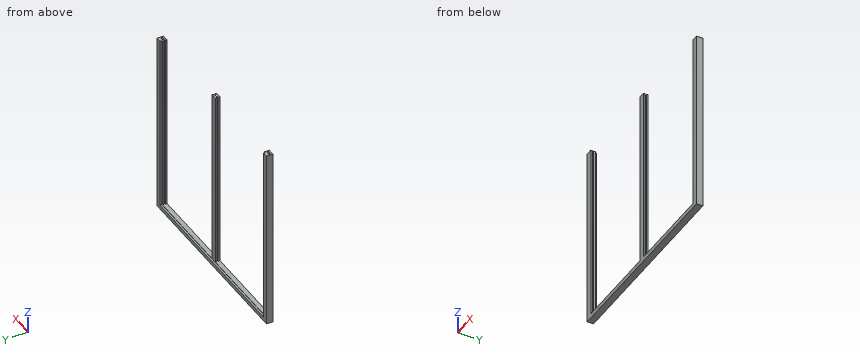
```python
from build123d import *

# Parameters (mm, degrees)
SKETCH1_W           = 2.25
SKETCH1_H           = 1.45
BOSS_EXTRUDE1_DEPTH = 5
BOSS_EXTRUDE2_DEPTH = 200
BOSS_EXTRUDE3_DEPTH = 2
SKETCH4_W           = 2
SKETCH4_H           = 2
CUT_EXTRUDE1_DEPTH  = 3


with BuildPart() as part:
    # Sketch1 → Boss-Extrude1 (new body)
    with BuildSketch(Plane.XY):
        Polygon((0, 0), (7, 0), (7, 1.775), (4.75, 1.775), (4.75, 3.225), (7, 3.225), (7, 5), (0, 5), align=None)
        with Locations((5.875, 2.5)):
            Rectangle(SKETCH1_W, SKETCH1_H)
        Polygon((7, 0), (102.75, 0), (102.75, 1.775), (102.75, 3.225), (102.75, 5), (7, 5), (7, 3.225), (7, 1.775), align=None)
        with Locations((103.875, 2.5)):
            Rectangle(SKETCH1_W, SKETCH1_H)
        Polygon((102.75, 0), (106, 0), (106, 5), (102.75, 5), (102.75, 3.225), (105, 3.225), (105, 1.775), (102.75, 1.775), align=None)
        Polygon((106, 5), (106, 0), (109.25, 0), (109.25, 1.775), (107, 1.775), (107, 3.225), (109.25, 3.225), (109.25, 5), align=None)
        with Locations((108.125, 2.5)):
            Rectangle(SKETCH1_W, SKETCH1_H)
        Polygon((109.25, 1.775), (109.25, 0), (205, 0), (205, 1.775), (205, 3.225), (205, 5), (109.25, 5), (109.25, 3.225), align=None)
        with Locations((206.125, 2.5)):
            Rectangle(SKETCH1_W, SKETCH1_H)
        Polygon((205, 1.775), (205, 0), (212, 0), (212, 5), (205, 5), (205, 3.225), (207.25, 3.225), (207.25, 1.775), align=None)
    extrude(amount=BOSS_EXTRUDE1_DEPTH)

    # Sketch2 → Boss-Extrude2 (add)
    with BuildSketch(Plane.XY.offset(5)):
        Polygon((7, 3.225), (7, 5), (0, 5), (0, 0), (7, 0), (7, 1.775), (4.75, 1.775), (4.75, 3.225), align=None)
        Polygon((109.25, 3.225), (109.25, 5), (102.75, 5), (102.75, 3.225), (105, 3.225), (105, 1.775), (102.75, 1.775), (102.75, 0), (109.25, 0), (109.25, 1.775), (107, 1.775), (107, 3.225), align=None)
        Polygon((205, 5), (205, 3.225), (207.25, 3.225), (207.25, 1.775), (205, 1.775), (205, 0), (212, 0), (212, 5), align=None)
    extrude(amount=BOSS_EXTRUDE2_DEPTH)

    # Sketch3 → Boss-Extrude3 (add)
    with BuildSketch(Plane(origin=(0, 5, 0), x_dir=(1, 0, 0), z_dir=(0, 1, 0))):
        Polygon((5.5, -205), (5.5, -4.5), (206.5, -4.5), (206.5, -205), (212, -205), (212, 0), (0, 0), (0, -205), align=None)
    extrude(amount=BOSS_EXTRUDE3_DEPTH)

    # Sketch4 → Cut-Extrude1 (cut)
    with BuildSketch(Plane.XY.offset(205)):
        with Locations((209.5, 2.76849414)):
            Rectangle(SKETCH4_W, SKETCH4_H)
        with Locations((2.5, 2.76849414)):
            Rectangle(SKETCH4_W, SKETCH4_H)
    extrude(amount=-CUT_EXTRUDE1_DEPTH, mode=Mode.SUBTRACT)


solid = part.part
```
Input: part model. Units: mm. Frame: model coordinates. Coordinates: 2 decimals unless noted, no trailing zeros. Loops run counter-clockwise (first coordinate to the right, second up) from the corner with the lowest first, then second, coordinate; pieces in that order, holes last.
Q1. Contact query for flat-ended pins moving along their axis: pin 1 (0.6 mm diameter, centred on x = 2, y = 2.5, fed in from +Z); pin 2 (1.8 mm diameter, centred on x = 103.5, z = 85.5, fed in from +Y); pin 3 (1 mm diameter, centred on x = 129, y = 3, fed in from +Z). Output: stop coordinate, or through.
Results are:
pin 1: stops at z = 202
pin 2: stops at y = 5
pin 3: stops at z = 5
Q2. Section B-B, the plane x = 123. Return the cut outline in (y, z), and give its area (3 significant figures).
Results are:
outline: (0, 0) - (7, 0) - (7, 4.5) - (5, 4.5) - (5, 5) - (0, 5) - close
area: 34.0 mm2
Q3. Line query: line 1 along X through (y, z) = (3, 105.5); line 2 along X through (y, z) = (1.5, 143); line 3 along X through (y, z) = (6, 29). Output: solid intervals per line, ascending.
Results are:
line 1: x = 0 to 4.75, 105 to 107, 207.25 to 212
line 2: x = 0 to 7, 102.75 to 109.25, 205 to 212
line 3: x = 0 to 5.5, 206.5 to 212
Q4. Section A-A, the plane z = 24. Give the number of separate pieces and of enclosed holes in the cut face, and give its area (3 significant figures).
Results are:
separate pieces: 3
enclosed holes: 0
area: 111 mm2
